Check sheet for the drawn part. Datum: minimum x, y, z corner. Units: mm. A direction names the side the tool comes from. Round coordinates to 2 decimals unless told otherwise and drop trailing zeros. Loops run counter-clockwise (first coordinate to the right, second up) from the corner with the lowest first, then second, coordinate; pieces in that order, holes last.
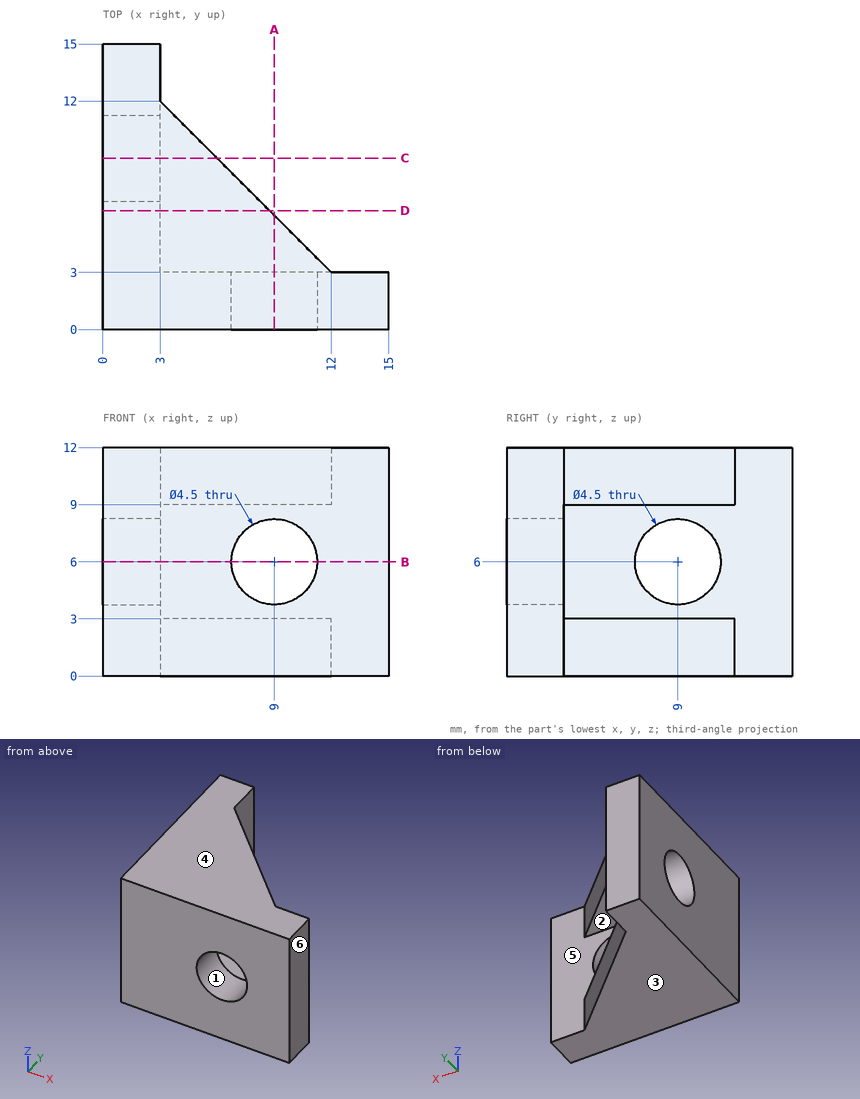
1. Section check D-D (y = 6.25). Enter the section's corners in (x, z).
2. Tool access check on the marked faces 1 and 2. Record the directions out of +Z, -Z, +X, -X, +Y, -Y that give a thin tool (end or side, any length) a straight path to the whole face; none if there is none.
3. Scan lines: L1, parallel to Y at x = 2.2, z = 6; L2, parallel to Z at x = 6, y = 3.25; L3, parallel to Z at x = 9, y = 2.05. Record each from-to range of solid material in increasing order.
4. Release check for a two-part mould opening along Z. For the marked faces 3, 4, 5 and 6 record: released by +Z, released by -Z, zero draft, split by the parting line, or undercut.
5. Section check B-B (z = 6). Enter the section's corners in (x, y).
6. Section check A-A (x = 9). Enter the section's corners in (y, z).
Taken from the geometry:
1. outline: (0, 0) - (8.75, 0) - (8.75, 3) - (3, 3) - (3, 9) - (8.75, 9) - (8.75, 12) - (0, 12) - close
2. face 1: +Y, -Y
2. face 2: +X, +Y
3. L1: y = 0 to 6.75, 11.25 to 15
3. L2: z = 0 to 3, 9 to 12
3. L3: z = 0 to 3.75, 8.25 to 12
4. face 3: released by -Z
4. face 4: released by +Z
4. face 5: undercut
4. face 6: zero draft
5. outline: (0, 0) - (6.75, 0) - (6.75, 3) - (3, 3) - (3, 6.75) - (0, 6.75) - close; (0, 11.25) - (3, 11.25) - (3, 15) - (0, 15) - close; (11.25, 0) - (15, 0) - (15, 3) - (11.25, 3) - close
6. outline: (0, 0) - (6, 0) - (6, 3) - (3, 3) - (3, 3.75) - (0, 3.75) - close; (0, 8.25) - (3, 8.25) - (3, 9) - (6, 9) - (6, 12) - (0, 12) - close
